from build123d import *

# Parameters (mm, degrees)
F0_W     = 114
F0_H     = 162
F1_DEPTH = 185
F3_DEPTH = 114
F5_W     = 109
F5_H     = 157
F6_DEPTH = 182.501


with BuildPart() as f1:
    # F0 (on Top) → F1 (new body)
    with BuildSketch(Plane.XY):
        with Locations((-57, -81)):
            Rectangle(F0_W, F0_H)
    extrude(amount=F1_DEPTH)

    # F2 (on Right) → F3 (cut, through all)
    with BuildSketch(Plane.YZ):
        Polygon((-162, 185), (-162, 50), (-159.5, 50), (-2.5, 185), align=None)
    extrude(amount=-F3_DEPTH, mode=Mode.SUBTRACT)

    # F5 (on offset) → F6 (cut, through all)
    with BuildSketch(Plane.XY.offset(2.5)):
        with Locations((-57, -81)):
            Rectangle(F5_W, F5_H)
    extrude(amount=F6_DEPTH, mode=Mode.SUBTRACT)


solid = f1.part
Design review of the part built by this model. Coordinates are the model's own, in mm. A direction names the side the tool comes from. Give positions to 0.01 mm unless a question says otherwise; leave off trailing zeros. Loops run counter-clockwise (first coordinate to the right, second up) from the corner with the lowest first, then second, coordinate; pieces in that order, holes last. Notation, with made-up numbers: M 40.25,84.5 L 84.25,84.5 A22 ccw 84.25,109.5 Z; hole C -5.5,-14.75 d10. An arc over 180 degrees is marked long. Answer as a JSON object with one key per item and string values.
Item 1: Mouldability with a two-part tool opening along Y and no side actions: class faces 1 (the face through (-58, -162, 25)), 2 (the face through (-58, -80, 0)), 3 (the face through (-58, -80, 2.5)) as pulls with the +Y half, pulls with the -Y half, needs draft (parallel to the pull), parting line crosses it, or undercut.
Output values:
{"face 1": "pulls with the -Y half", "face 2": "needs draft", "face 3": "undercut"}
Item 2: We need section B-B (x = -52.5). State the section outline as (y, z) points.
Output values:
{"outline": "M -162,0 L 0,0 L 0,185 L -2.5,185 L -2.5,2.5 L -159.5,2.5 L -159.5,50 L -162,50 Z"}
Item 3: We need section A-A (z = 32). State the section outline as (x, y) points, and give its area (4 significant figures).
Output values:
{"outline": "M -114,-162 L 0,-162 L 0,0 L -114,0 Z; hole M -111.5,-159.5 L -2.5,-159.5 L -2.5,-2.5 L -111.5,-2.5 Z", "area": "1,355 mm2"}
Item 4: Wall thickness on line 1 along Y through (x, z) = (-107.5, 17); line 2 along X through (y, z) = (-65, 86); line 3 along Z through (x, y) = (-77.5, -59.5): over which ranges is each line inside the solid? List them lowest first.
Output values:
{"line 1": "y = -162 to -159.5, -2.5 to 0", "line 2": "x = -114 to -111.5, -2.5 to 0", "line 3": "z = 0 to 2.5"}
Item 5: We need section C-C (y = -134). State the section outline as (x, z) points.
Output values:
{"outline": "M -114,0 L 0,0 L 0,71.93 L -2.5,71.93 L -2.5,2.5 L -111.5,2.5 L -111.5,71.93 L -114,71.93 Z"}
Item 6: For P1, Ø1.5, axis at x = -89.5, y = -143, coming from the +Z side; P2, Ø1.5, axis at x = -56, z = 76, coming from the -Y side; P3, Ø1.2, axis at x = -79.5, y = -161, coming from the +Z side, all flat-tipped, find the tip position at first contact; note any pin that passes through.
Output values:
{"P1": "stops at z = 2.5", "P2": "stops at y = -2.5", "P3": "stops at z = 50"}
Item 7: Machinability: for faces 4 (the face through (-111.5, -65, 72)), 5 (the face through (0, -64, 71)), which of the approach directions +Z, -Z, +X, -X, +Y, -Y give a long, thin tool a straight path to every point of the face, cutting with its end or side? Answer none if there is none.
Output values:
{"face 4": "+Z", "face 5": "+Z, -Z, +X, +Y, -Y"}
